Answer from the drawing. Dimensions are ordinates in mm from the lowest x, y and z of the part. A direction names the side the tool comes from. Round coordinates to 2 decimals unless told otherwise and drop trailing zeros. Loops run counter-clockwise (first coordinate to the right, second up) from the corner with the lowest first, then second, coordinate; pieces in that order, holes last. Notation, with made-up numbers: M -31.75,6.5 L 0.25,6.5 A24 ccw 0.25,40.5 Z; hole C -14.5,48.25 d2. An arc over 180 degrees is marked long. One line per item, written item: value.
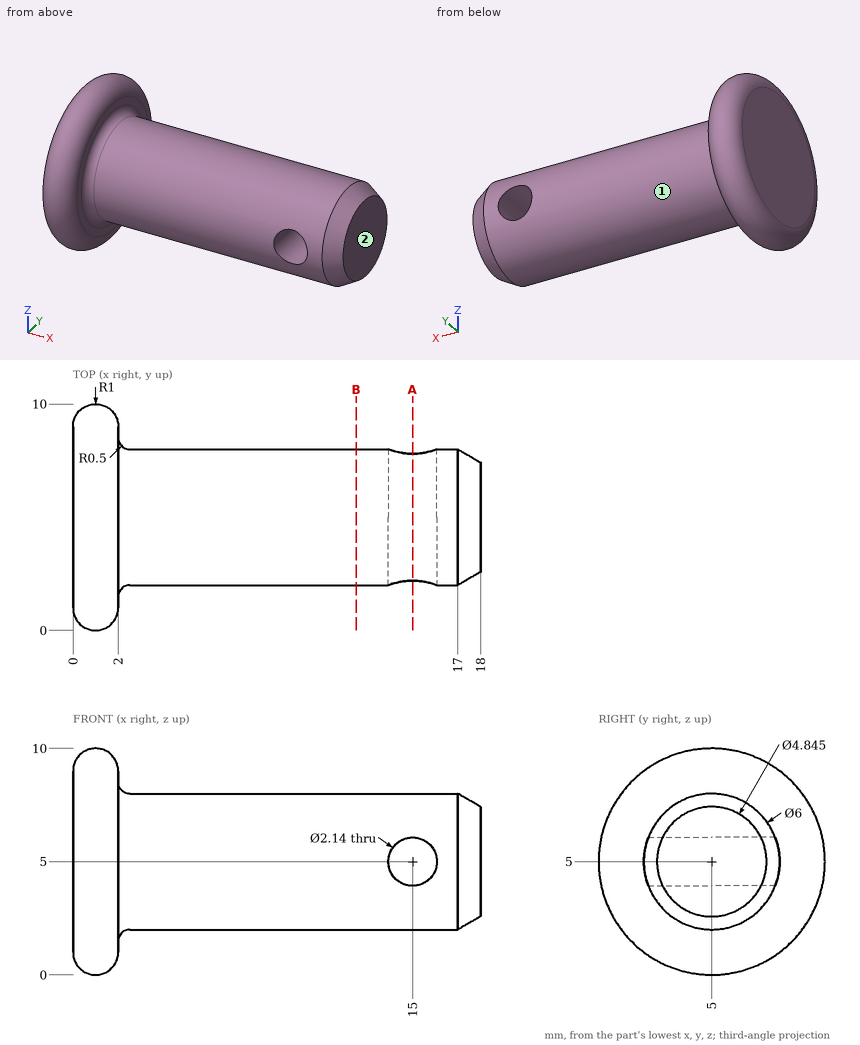
1) Find section B-B (x = 12.5). Give the vertices of the cut face in (y, z), then the cut area to 3 significant figures.
Check values:
outline: C 5,5 d6
area: 28.3 mm2
2) Find section A-A (x = 15). Give the vertices of the cut face in (y, z), then the cut area to 3 significant figures.
Check values:
outline: M 2.2,3.93 A3 ccw 7.8,3.93 Z; M 2.2,6.07 L 7.8,6.07 A3 ccw Z
area: 15.7 mm2
3) For the marked faces 1 and 2, determine the directions among +Z, -Z, +X, -X, +Y, -Y from which every point of the face is accessible in a straight line to the end or side of a thin tool.
Check values:
face 1: +X
face 2: +Z, -Z, +X, +Y, -Y
4) Find the intervals of material crossed by probe 1 along X at (y, z) = (5.25, 8.5); probe 2 along Z at (x, y) = (15, 6.55); probe 3 along Z at (x, y) = (15, 6.6), in increasing order. Write a range as from..to.
Check values:
probe 1: 0..2
probe 2: 2.43..3.93, 6.07..7.57
probe 3: 2.46..3.93, 6.07..7.54
5) Each of these flat-tipped pins is pushed along its axis until it touches: pin 1 (5 mm diameter, centred on x = 7.5, z = 4, fed in from +Y); pin 2 (6 mm diameter, centred on x = 5.5, z = 6.5, fed in from -Y); pin 3 (4 mm diameter, centred on x = 2.5, y = 3, fed in from +Z). Where does it stop, or does it pass through?
Check values:
pin 1: y = 8
pin 2: y = 2
pin 3: z = 9.96
